Model file for the job. Use its own axes, mm. Face numbers are marked on the shaded views. A direction names the side the tool comes from. Round coordinates to 2 decimals unless told otherwise and drop trailing zeros. Loops run counter-clockwise (first coordinate to the right, second up) from the corner with the lowest first, then second, coordinate; pieces in that order, holes last. Notation, with made-up numbers: (33.25, 80.25) - (39.25, 80.25) arc R20 ccw to (39.25, 104.25) - close; hole circle Ø10 at (2, 38). An arc over 180 degrees is marked (long way). Answer as a JSON object with one key per item and string values.
from build123d import *

# Parameters (mm, degrees)
SKETCH2_W           = 3
SKETCH2_H           = 2
CHAMFER1_SIZE       = 2
CUT_EXTRUDE1_DEPTH  = 132.057239403
CIRPATTERN1_COUNT   = 3
HOLE1_D             = 12
CIRPATTERN2_COUNT   = 3
CUT_EXTRUDE2_START  = -79
CUT_EXTRUDE2_DEPTH  = 79
BOSS_EXTRUDE2_START = -19
SKETCH9_R           = 41
BOSS_EXTRUDE2_DEPTH = 19
HOLE3_D             = 19
HOLE3_CBORE_D       = 44
HOLE3_CBORE_DEPTH   = 4


with BuildPart() as part:
    # Sketch1 → Revolve3 (revolve)
    with BuildSketch(Plane.XY, mode=Mode.PRIVATE) as revolve3_sk:
        Polygon((0, 0), (0, 66), (14, 66), (14, 41), (19, 41), (19, 17.5), (84, 17.5), (84, 12.5), (106, 12.5), (106, 0), align=None)
    revolve(revolve3_sk.sketch.rotate(Axis((0, 0, 0), (1, 0, 0)), 90), axis=Axis((0, 0, 0), (1, 0, 0)))

    # Sketch2 → Cut-Revolve1 (revolve, cut)
    with BuildSketch(Plane.XY, mode=Mode.PRIVATE) as cut_revolve1_sk:
        with Locations((85.5, 11.5)):
            Rectangle(SKETCH2_W, SKETCH2_H)
    revolve(cut_revolve1_sk.sketch.rotate(Axis((0, 0, 0), (1, 0, 0)), 90), axis=Axis((0, 0, 0), (1, 0, 0)), mode=Mode.SUBTRACT)

    # Sketch3 → Revolve5 (revolve)
    with BuildSketch(Plane(origin=(0, 0, 0), x_dir=(1, 0, 0), z_dir=(0, 1, 0)), mode=Mode.PRIVATE) as revolve5_sk:
        Polygon((19, 36.5), (82, 17.5), (19, 17.5), align=None)
    revolve(revolve5_sk.sketch.rotate(Axis((0, 0, 0), (1, 0, 0)), 180), axis=Axis((0, 0, 0), (1, 0, 0)))

    # Chamfer1
    chamfer1_edges = [part.edges().sort_by_distance(p)[0] for p in [
        (106, 0, -12.5),
        (84, 0, -17.5),
    ]]
    chamfer(chamfer1_edges, length=CHAMFER1_SIZE - 0.0001)  # a hair under: the kernel refuses the full size

    # Sketch4 → Cut-Extrude1 (cut, through all)
    with BuildSketch(Plane(origin=(14, 0, 0), x_dir=(0, 0, -1), z_dir=(1, 0, 0))):
        with BuildLine():
            Line((-32.5, -57.443450453), (-25, -44.453069397))
            Line((-25, -44.453069397), (25, -44.453069397))
            Line((25, -44.453069397), (32.5, -57.443450453))
            ThreePointArc((32.5, -57.443450453), (0, -66), (-32.5, -57.443450453))
        make_face()
    cut_extrude1 = extrude(amount=-CUT_EXTRUDE1_DEPTH, mode=Mode.SUBTRACT)

    # CirPattern1: Cut-Extrude1 ×3 about axis
    cirpattern1_axis = Axis((0, 0, 0), (1, 0, 0))
    for i in range(1, CIRPATTERN1_COUNT):
        add(cut_extrude1.rotate(cirpattern1_axis, i * 360 / CIRPATTERN1_COUNT), mode=Mode.SUBTRACT)

    # Hole1 (through all)
    with Locations(Plane(origin=(14, 0, 0), x_dir=(0, 0, -1), z_dir=(1, 0, 0))):
        with Locations((0, 53.5)):
            hole1 = Hole(HOLE1_D / 2)

    # CirPattern2: Hole1 ×3 about axis
    cirpattern2_axis = Axis((0, 0, 0), (1, 0, 0))
    for i in range(1, CIRPATTERN2_COUNT):
        add(hole1.rotate(cirpattern2_axis, i * 360 / CIRPATTERN2_COUNT), mode=Mode.SUBTRACT)

    # Sketch7 → Cut-Extrude2 (cut)
    with BuildSketch(Plane.ZY.offset(CUT_EXTRUDE2_START)):
        with BuildLine():
            Line((17.320508076, 2.5), (40.923709509, 2.5))
            ThreePointArc((40.923709509, 2.5), (35.507041555, 20.5), (22.626918264, 34.190972052))
            Line((22.626918264, 34.190972052), (10.825317547, 13.75))
            ThreePointArc((10.825317547, 13.75), (15.155444566, 8.75), (17.320508076, 2.5))
        make_face()
        with BuildLine():
            Line((17.320508076, -2.5), (40.923709509, -2.5))
            ThreePointArc((40.923709509, -2.5), (35.507041555, -20.5), (22.626918264, -34.190972052))
            Line((22.626918264, -34.190972052), (10.825317547, -13.75))
            ThreePointArc((10.825317547, -13.75), (15.155444566, -8.75), (17.320508076, -2.5))
        make_face()
        with BuildLine():
            Line((6.495190528, -16.25), (18.296791245, -36.690972052))
            ThreePointArc((18.296791245, -36.690972052), (0, -41), (-18.296791245, -36.690972052))
            Line((-18.296791245, -36.690972052), (-6.495190528, -16.25))
            ThreePointArc((-6.495190528, -16.25), (0, -17.5), (6.495190528, -16.25))
        make_face()
        with BuildLine():
            Line((-10.825317547, -13.75), (-22.626918264, -34.190972052))
            ThreePointArc((-22.626918264, -34.190972052), (-35.507041555, -20.5), (-40.923709509, -2.5))
            Line((-40.923709509, -2.5), (-17.320508076, -2.5))
            ThreePointArc((-17.320508076, -2.5), (-15.155444566, -8.75), (-10.825317547, -13.75))
        make_face()
        with BuildLine():
            Line((-17.320508076, 2.5), (-40.923709509, 2.5))
            ThreePointArc((-40.923709509, 2.5), (-35.507041555, 20.5), (-22.626918264, 34.190972052))
            Line((-22.626918264, 34.190972052), (-10.825317547, 13.75))
            ThreePointArc((-10.825317547, 13.75), (-15.155444566, 8.75), (-17.320508076, 2.5))
        make_face()
        with BuildLine():
            Line((-6.495190528, 16.25), (-18.296791245, 36.690972052))
            ThreePointArc((-18.296791245, 36.690972052), (0, 41), (18.296791245, 36.690972052))
            Line((18.296791245, 36.690972052), (6.495190528, 16.25))
            ThreePointArc((6.495190528, 16.25), (0, 17.5), (-6.495190528, 16.25))
        make_face()
    extrude(amount=CUT_EXTRUDE2_DEPTH, mode=Mode.SUBTRACT)

    # Sketch9 → Boss-Extrude2 (add)
    with BuildSketch(Plane.ZY.offset(BOSS_EXTRUDE2_START)):
        Circle(SKETCH9_R)
    extrude(amount=BOSS_EXTRUDE2_DEPTH)

    # Hole3 (through all)
    with Locations(Plane.ZY):
        with Locations((0, 0)):
            CounterBoreHole(HOLE3_D / 2, HOLE3_CBORE_D / 2, HOLE3_CBORE_DEPTH)


solid = part.part
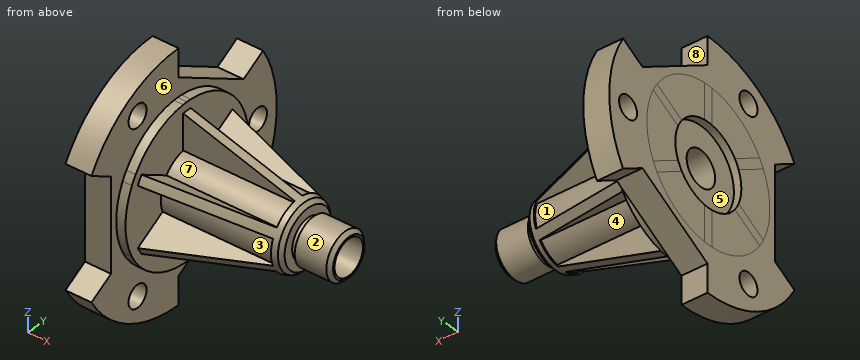
1) Slice it at D-D on y = -27. Count the separate pieces of the cut face and the enclosed holes in it, then the cut area to 3 significant figures.
Values follow:
{"separate pieces": "3", "enclosed holes": "0", "area": "1,860 mm²"}
2) Slice it at B-B on y = 53.5. List the corners of the cut face in (x, z), then the cut area to 3 significant figures.
Values follow:
{"outline": "(0, -31.55) - (14, -31.55) - (14, -6) - (0, -6) - close; (0, 6) - (14, 6) - (14, 31.55) - (0, 31.55) - close", "area": "715 mm²"}
3) Drop flat-ended pins along their axis: P1, Ø1, axis at y = -10, z = 19, coming from the +X side; P2, Ø0.6, axis at y = 17, z = 2.5, coming from the -X side; P3, Ø15.5, axis at x = 59.5, z = -26.5, coming from the -Y side; P4, Ø11, axis at y = 53.5, z = 0, coming from the -X side. Give the stop position or say it passes through.
Values follow:
{"P1": "x = 19", "P2": "x = 4", "P3": "y = -2.5", "P4": "through"}
4) Slice it at A-A on x = 64. List the corners of the cut face in (y, z), then the cut area to 3 significant figures.
Values follow:
{"outline": "(-20.99, -9.23) arc R22.93 ccw to (-18.49, -13.56) - (-13.75, -10.83) arc R17.5 ccw to (-2.5, -17.32) - (-2.5, -22.79) arc R22.93 ccw to (2.5, -22.79) - (2.5, -17.32) arc R17.5 ccw to (13.75, -10.83) - (18.49, -13.56) arc R22.93 ccw to (20.99, -9.23) - (16.25, -6.5) arc R17.5 ccw to (16.25, 6.5) - (20.99, 9.23) arc R22.93 ccw to (18.49, 13.56) - (13.75, 10.83) arc R17.5 ccw to (2.5, 17.32) - (2.5, 22.79) arc R22.93 ccw to (-2.5, 22.79) - (-2.5, 17.32) arc R17.5 ccw to (-13.75, 10.83) - (-18.49, 13.56) arc R22.93 ccw to (-20.99, 9.23) - (-16.25, 6.5) arc R17.5 ccw to (-16.25, -6.5) - close; hole circle Ø19 at (0, 0)", "area": "842 mm²"}
5) Two-plate mould, pull along Y, no slides. Class the marked faces 6, 7 and 8: pulls with the +Y half, pulls with the -Y half, needs draft (parallel to the pull), parting line crosses it, or undercut.
Values follow:
{"face 6": "needs draft", "face 7": "undercut", "face 8": "pulls with the +Y half"}
6) Probe probe 1 along Y at (x, z) = (1, 0); probe 2 along Y at (x, z) = (59, -12); probe 3 along X at (y, z) = (-38.5, -5). List the from-to ranges inside material, lowest first.
Values follow:
{"probe 1": "-44.45 to -22, 22 to 47.5, 59.5 to 66", "probe 2": "-21.29 to -15.78, -12.74 to 12.74, 15.78 to 21.29", "probe 3": "0 to 19"}
7) Slice it at C-C on z = 47.5. List the corners of the cut face in (x, y), then the cut area to 3 significant figures.
Values follow:
{"outline": "(0, -45.82) - (14, -45.82) - (14, -32.64) - (0, -32.64) - close; (0, -20.86) - (14, -20.86) - (14, 6.63) - (0, 6.63) - close", "area": "570 mm²"}
8) Tool access for the marked faces 1, 2, 3, 4 and 5: list every direction of +Z, -Z, +X, -X, +Y, -Y with a clear straight run to the whole face (end or side of a thin tool).
Values follow:
{"face 1": "+Y", "face 2": "+X", "face 3": "-Y", "face 4": "-Z", "face 5": "-X"}
